from build123d import *

# Parameters (mm, degrees)
SKETCH1_R           = 9.5
BOSS_EXTRUDE1_DEPTH = 2.5
SKETCH2_R           = 7.9
BOSS_EXTRUDE2_DEPTH = 8.2
SKETCH3_R           = 9.5
BOSS_EXTRUDE3_DEPTH = 2.5
SKETCH4_R           = 4.45
SKETCH4_W           = 10.190914757
SKETCH4_H           = 1.75
CUT_EXTRUDE1_DEPTH  = 19.834542734


with BuildPart() as part:
    # Sketch1 → Boss-Extrude1 (new body)
    with BuildSketch(Plane(origin=(0, 0, 0), x_dir=(1, 0, 0), z_dir=(0, 1, 0))):
        with Locations(Location((0, 0, 0), (0, 0, 270))):
            Circle(SKETCH1_R)
    extrude(amount=BOSS_EXTRUDE1_DEPTH)

    # Sketch2 → Boss-Extrude2 (add)
    with BuildSketch(Plane(origin=(0, 2.5, 0), x_dir=(1, 0, 0), z_dir=(0, 1, 0))):
        with Locations(Location((0, 0, 0), (0, 0, 270))):
            Circle(SKETCH2_R)
    extrude(amount=BOSS_EXTRUDE2_DEPTH)

    # Sketch3 → Boss-Extrude3 (add)
    with BuildSketch(Plane(origin=(0, 10.7, 0), x_dir=(1, 0, 0), z_dir=(0, 1, 0))):
        with Locations(Location((0, 0, 0), (0, 0, 270))):
            Circle(SKETCH3_R)
    extrude(amount=BOSS_EXTRUDE3_DEPTH)

    # Sketch4 → Cut-Extrude1 (cut, through all)
    with BuildSketch(Plane(origin=(0, 13.2, 0), x_dir=(1, 0, 0), z_dir=(0, 1, 0))):
        Circle(SKETCH4_R)
        with Locations((5.901899369, 0)):
            Rectangle(SKETCH4_W, SKETCH4_H)
    extrude(amount=-CUT_EXTRUDE1_DEPTH, mode=Mode.SUBTRACT)


solid = part.part
Input: part model. Units: mm. Frame: model coordinates. A direction names the side the tool comes from. Coordinates: 2 decimals unless noted, no trailing zeros. Loops run counter-clockwise (first coordinate to the right, second up) from the corner with the lowest first, then second, coordinate; pieces in that order, holes last. Notation, with made-up numbers: (31.5, 56) -> (42.5, 56) arc R21 ccw to (42.5, 74) -> close; hole circle Ø7 at (73, 83). An arc over 180 degrees is marked (long way). Write item = value, one per line. Start each with the question number.
Item 1: Cut plane C-C, the plane z = 5.5. Return loops of the section in (x, y).
Item 2: Cut plane B-B, the plane z = -1.5. Return loops of the section in (x, y).
Item 3: Cut plane D-D, the plane y = 6.75. Return loops of the section in (x, z) (3 decimals).
Item 4: Cut plane A-A, the plane x = 0. Return loops of the section in (y, z), plus the area to 3 significant figures.
Item 5: Mould query, pull axis Z, two halves, no side actions, for faces 4 (the face through (-7.893, 6.543, -0.335)), 5 (the face through (6, 7, -0.875)), 6 (the face through (-4.1, 0, -2.2)). Classes: pulls with the +Z half, pulls with the -Z half, needs draft (parallel to the pull), parting line crosses it, or undercut.
Item 6: First-contact query: P1, Ø3, axis at y = 6.5, z = 5, coming from the -X side; P2, Ø1.5, axis at x = 7, y = 6, coming from the -Z side; P3, Ø2.5, axis at x = 6, y = 5, coming from the +Z side. Flat tips, straight axial feed; report the tip coordinate or a pass-through.
Item 7: Reachability of faces 1 (the face through (-4.446, 6.692, -0.183)), 2 (the face through (6, 7, 0.875)), 3 (the face through (-6, 10.7, -6)) from +Z, -Z, +X, -X, +Y, -Y: full face, straight path, thin tool, end or side. Return the list, or none.
Item 8: Material intervals for line 1 (Z direction, x = 0, y = 4.5); line 2 (Y direction, x = -8.25, z = -3.5); line 3 (Z direction, x = 4.5, y = 2.25) (3 decimals), sorted ascending.
Ans:
q1.outline = (-7.75, 0) -> (7.75, 0) -> (7.75, 2.5) -> (5.67, 2.5) -> (5.67, 10.7) -> (7.75, 10.7) -> (7.75, 13.2) -> (-7.75, 13.2) -> (-7.75, 10.7) -> (-5.67, 10.7) -> (-5.67, 2.5) -> (-7.75, 2.5) -> close
q2.outline = (-9.38, 0) -> (-4.19, 0) -> (-4.19, 13.2) -> (-9.38, 13.2) -> (-9.38, 10.7) -> (-7.76, 10.7) -> (-7.76, 2.5) -> (-9.38, 2.5) -> close; (4.19, 0) -> (9.38, 0) -> (9.38, 2.5) -> (7.76, 2.5) -> (7.76, 10.7) -> (9.38, 10.7) -> (9.38, 13.2) -> (4.19, 13.2) -> close
q3.outline = (4.363, -0.875) arc R4.45 cw (long way) to (4.363, 0.875) -> (7.851, 0.875) arc R7.9 ccw (long way) to (7.851, -0.875) -> close
q4.outline = (0, -9.5) -> (2.5, -9.5) -> (2.5, -7.9) -> (10.7, -7.9) -> (10.7, -9.5) -> (13.2, -9.5) -> (13.2, -4.45) -> (0, -4.45) -> close; (0, 4.45) -> (13.2, 4.45) -> (13.2, 9.5) -> (10.7, 9.5) -> (10.7, 7.9) -> (2.5, 7.9) -> (2.5, 9.5) -> (0, 9.5) -> close
q4.area = 107 mm²
q5.face_4 = parting line crosses it
q5.face_5 = undercut
q5.face_6 = needs draft
q6.P1 = -7.08
q6.P2 = -4.83
q6.P3 = 6.31
q7.face_1 = +Y, -Y
q7.face_2 = +X, +Y, -Y
q7.face_3 = none
q8.line_1 = -7.9 to -4.45, 4.45 to 7.9
q8.line_2 = 0 to 2.5, 10.7 to 13.2
q8.line_3 = -8.367 to -0.875, 0.875 to 8.367
